from build123d import *

# Parameters (mm, degrees)
BOSS_EXTRUDE1_START = 4.7625
SKETCH3_R           = 11.1125
SKETCH3_R_2         = 6.3627
BOSS_EXTRUDE1_DEPTH = 3.175
BOSS_EXTRUDE2_START = 1.5875
SKETCH4_R           = 7.9629
SKETCH4_R_2         = 6.3627
BOSS_EXTRUDE2_DEPTH = 6.35
CHAMFER1_SIZE       = 0.190881


with BuildPart() as part:
    # Sketch3 → Boss-Extrude1 (new body)
    with BuildSketch(Plane.XY.offset(BOSS_EXTRUDE1_START)):
        Circle(SKETCH3_R)
        Circle(SKETCH3_R_2, mode=Mode.SUBTRACT)
    extrude(amount=-BOSS_EXTRUDE1_DEPTH)

    # Sketch4 → Boss-Extrude2 (add)
    with BuildSketch(Plane.XY.offset(BOSS_EXTRUDE2_START)):
        Circle(SKETCH4_R)
        Circle(SKETCH4_R_2, mode=Mode.SUBTRACT)
    extrude(amount=-BOSS_EXTRUDE2_DEPTH)

    # Chamfer1
    chamfer1_edges = [part.edges().sort_by_distance(p)[0] for p in [
        (-6.3627, 0, -4.7625),
        (-7.9629, 0, 1.5875),
        (-11.1125, 0, 4.7625),
        (-11.1125, 0, 1.5875),
        (-6.3627, 0, 4.7625),
        (-7.9629, 0, -4.7625),
    ]]
    chamfer(chamfer1_edges, length=CHAMFER1_SIZE)


solid = part.part
Read the model definition and answer for the solid it produces. Units are mm, in the model's axes. A direction names the side the tool comes from. Give positions to 0.01 mm unless a question says otherwise; leave off trailing zeros. Write each loop counter-clockwise with the first axis right and the second up, starting at its lowest first coordinate (ties: lowest second). Pieces come first, ordered by that corner, then holes. Notation, with made-up numbers: (21.5, -5.5) - (80.5, -5.5) arc R25 cw to (80.5, 20.5) - close; hole circle Ø5 at (-33.5, -29). An arc over 180 degrees is marked (long way). Answer in a Markdown table with one row per item. Add a question column.
Item 1: Section D-D, the plane z = -0.5 is taken. Write down the section's boundary in (x, y).
Item 2: Section C-C, the plane z = 3 is taken. Write down the section's boundary in (x, y) (1 decimal), and give its area (3 significant figures).
Item 3: Section A-A, the plane y = 0 is taken. Write down the section's boundary in (x, z).
Item 4: Find the intervals of material crossed by L1, parallel to Y at x = 0, z = -1.25; L2, parallel to Y at x = 0, z = 2, in increasing order.
Item 5: Determine the mould class of faces 3 (the face through (-0.83, 6.31, 0.06)), 4 (the face through (5, -5, 4.762)), 5 (the face through (10.6, 3.34, 3.19)) for opening direction X: pulls with the +X half, pulls with the -X half, needs draft (parallel to the pull), parting line crosses it, or undercut.
Item 6: Flat-ended cylindrical pins translate along their axes: P1, Ø1.5, axis at y = 1, z = -3, coming from the +X side; P2, Ø1.5, axis at x = -7.5, z = 2, coming from the -Y side; P3, Ø1, axis at x = -6.5, z = 1, coming from the -Y side; P4, Ø2, axis at x = -3, y = 3.5, coming from the +Z side. Find the tip coordinate at first contact, or state that the pin passes through.
Item 7: A tool of negligible diameter and unlimited length cuts with its end or side. For faces 1 (the face through (-4.1, -7.23, 1.588)), 2 (the face through (-3, -6, -4.762)), from which of +Z, -Z, +X, -X, +Y, -Y can it reach the whole face along a straight path? Write none if from no direction.
Recorded:
| question | item | result |
|---|---|---|
| 1 | outline | circle Ø15.93 at (0, 0); hole circle Ø12.73 at (0, 0) |
| 2 | outline | circle Ø22.2 at (0, 0); hole circle Ø12.7 at (0, 0) |
| 2 | area | 261 mm2 |
| 3 | outline | (-11.11, 1.78) - (-10.92, 1.59) - (-8.15, 1.59) - (-7.96, 1.4) - (-7.96, -4.57) - (-7.77, -4.76) - (-6.55, -4.76) - (-6.36, -4.57) - (-6.36, 4.57) - (-6.55, 4.76) - (-10.92, 4.76) - (-11.11, 4.57) - close; (6.36, -4.57) - (6.55, -4.76) - (7.77, -4.76) - (7.96, -4.57) - (7.96, 1.4) - (8.15, 1.59) - (10.92, 1.59) - (11.11, 1.78) - (11.11, 4.57) - (10.92, 4.76) - (6.55, 4.76) - (6.36, 4.57) - close |
| 4 | L1 | y = -7.96 to -6.36, 6.36 to 7.96 |
| 4 | L2 | y = -11.11 to -6.36, 6.36 to 11.11 |
| 5 | face 3 | undercut |
| 5 | face 4 | needs draft |
| 5 | face 5 | parting line crosses it |
| 6 | P1 | stops at x = 7.96 |
| 6 | P2 | stops at y = -8.83 |
| 6 | P3 | stops at y = -5.24 |
| 6 | P4 | passes through |
| 7 | face 1 | -Z |
| 7 | face 2 | -Z, +X, -X, +Y, -Y |
